```python
from build123d import *

# Parameters (mm, degrees)
CROQUIS1_R              = 4
SALIENTE_EXTRUIR1_DEPTH = 171
CROQUIS2_R              = 17.5
SALIENTE_EXTRUIR2_DEPTH = 3
SALIENTE_EXTRUIR3_DEPTH = 5
CROQUIS4_R              = 4
SALIENTE_EXTRUIR4_DEPTH = 4.5
CROQUIS8_R              = 17.5
SALIENTE_EXTRUIR6_DEPTH = 3


with BuildPart() as part:
    # Croquis1 → Saliente-Extruir1 (new body)
    with BuildSketch(Plane(origin=(0, 0, 0), x_dir=(1, 0, 0), z_dir=(0, 1, 0))):
        Circle(CROQUIS1_R)
    extrude(amount=SALIENTE_EXTRUIR1_DEPTH)

    # Croquis2 → Saliente-Extruir2 (add)
    with BuildSketch(Plane(origin=(0, 29.389431256, -17.658951857), x_dir=(-1, 0, 0), z_dir=(0, -0.857167301, 0.515038075))):
        with Locations((0, -20.601522996)):
            Circle(CROQUIS2_R)
    extrude(amount=SALIENTE_EXTRUIR2_DEPTH)

    # Croquis3 → Saliente-Extruir3 (add)
    with BuildSketch(Plane(origin=(0, 171, 0), x_dir=(1, 0, 0), z_dir=(0, 1, 0))):
        with BuildLine():
            Line((1.050742858, 12.216507919), (0.472845286, 10.71499343))
            ThreePointArc((0.472845286, 10.71499343), (0, 10.543875222), (-0.472845286, 10.71499343))
            Line((-0.472845286, 10.71499343), (-1.050742858, 12.216507919))
            ThreePointArc((-1.050742858, 12.216507919), (-1.656207782, 12.14924286), (-2.257584572, 12.051988972))
            Line((-2.257584572, 12.051988972), (-2.426564451, 10.457781423))
            ThreePointArc((-2.426564451, 10.457781423), (-2.771930057, 10.239934406), (-3.179948954, 10.255912654))
            Line((-3.179948954, 10.255912654), (-4.120766374, 11.54843759))
            ThreePointArc((-4.120766374, 11.54843759), (-4.690827714, 11.328868507), (-5.249245828, 11.081179745))
            Line((-5.249245828, 11.081179745), (-5.000525386, 9.501805204))
            ThreePointArc((-5.000525386, 9.501805204), (-5.277739988, 9.201993948), (-5.675991453, 9.111824689))
            Line((-5.675991453, 9.111824689), (-6.923284582, 10.120042336))
            ThreePointArc((-6.923284582, 10.120042336), (-7.417219229, 9.763809974), (-7.892857245, 9.383492462))
            Line((-7.892857245, 9.383492462), (-7.239355878, 7.912212973))
            ThreePointArc((-7.239355878, 7.912212973), (-7.429527758, 7.55086912), (-7.790871612, 7.360697239))
            Line((-7.790871612, 7.360697239), (-9.275101788, 8.019950942))
            ThreePointArc((-9.275101788, 8.019950942), (-9.658562641, 7.553760256), (-10.018615343, 7.069262543))
            Line((-10.018615343, 7.069262543), (-8.990483327, 5.797332815))
            ThreePointArc((-8.990483327, 5.797332815), (-9.080652586, 5.39908135), (-9.380463842, 5.121866748))
            Line((-9.380463842, 5.121866748), (-11.018384727, 5.379807088))
            ThreePointArc((-11.018384727, 5.379807088), (-11.266454067, 4.838815873), (-11.487980236, 4.286424664))
            Line((-11.487980236, 4.286424664), (-10.134571292, 3.301290316))
            ThreePointArc((-10.134571292, 3.301290316), (-10.118593045, 2.893271419), (-10.336440061, 2.547905812))
            Line((-10.336440061, 2.547905812), (-12.0307187, 2.368318783))
            ThreePointArc((-12.0307187, 2.368318783), (-12.129855039, 1.792691558), (-12.201465745, 1.212996274))
            Line((-12.201465745, 1.212996274), (-10.593652069, 0.594186647))
            ThreePointArc((-10.593652069, 0.594186647), (-10.472615206, 0.204206132), (-10.593652069, -0.185774383))
            Line((-10.593652069, -0.185774383), (-12.234346993, -0.817239228))
            ThreePointArc((-12.234346993, -0.817239228), (-12.183011813, -1.386127504), (-12.105238209, -1.952007737))
            Line((-12.105238209, -1.952007737), (-10.336440061, -2.139493548))
            ThreePointArc((-10.336440061, -2.139493548), (-10.118593045, -2.484859155), (-10.134571292, -2.892878051))
            Line((-10.134571292, -2.892878051), (-11.603765461, -3.962291436))
            ThreePointArc((-11.603765461, -3.962291436), (-11.411733847, -4.485471759), (-11.196127365, -4.999385795))
            Line((-11.196127365, -4.999385795), (-9.380463842, -4.713454484))
            ThreePointArc((-9.380463842, -4.713454484), (-9.080652586, -4.990669086), (-8.990483327, -5.388920551))
            Line((-8.990483327, -5.388920551), (-10.170571543, -6.848839375))
            ThreePointArc((-10.170571543, -6.848839375), (-9.857154436, -7.29271093), (-9.524379813, -7.722261033))
            Line((-9.524379813, -7.722261033), (-7.790871612, -6.952284975))
            ThreePointArc((-7.790871612, -6.952284975), (-7.429527758, -7.142456856), (-7.239355878, -7.503800709))
            Line((-7.239355878, -7.503800709), (-8.024406446, -9.271247353))
            ThreePointArc((-8.024406446, -9.271247353), (-7.61599094, -9.60956858), (-7.193327687, -9.929912542))
            Line((-7.193327687, -9.929912542), (-5.675991453, -8.703412424))
            ThreePointArc((-5.675991453, -8.703412424), (-5.277739988, -8.793581684), (-5.000525386, -9.09339294))
            Line((-5.000525386, -9.09339294), (-5.309068741, -11.052642915))
            ThreePointArc((-5.309068741, -11.052642915), (-4.836465093, -11.26746341), (-4.355191926, -11.462086615))
            Line((-4.355191926, -11.462086615), (-3.179948954, -9.84750039))
            ThreePointArc((-3.179948954, -9.84750039), (-2.771930057, -9.831522142), (-2.426564451, -10.049369159))
            Line((-2.426564451, -10.049369159), (-2.213426541, -12.060176999))
            ThreePointArc((-2.213426541, -12.060176999), (-1.70946512, -12.141863749), (-1.202540078, -12.202500713))
            Line((-1.202540078, -12.202500713), (-0.472845286, -10.306581166))
            ThreePointArc((-0.472845286, -10.306581166), (-0.08286477, -10.185544303), (0.307115745, -10.306581166))
            Line((0.307115745, -10.306581166), (1.042474215, -12.217216287))
            ThreePointArc((1.042474215, -12.217216287), (1.544818551, -12.163908169), (2.04454079, -12.08995365))
            Line((2.04454079, -12.08995365), (2.26083491, -10.049369159))
            ThreePointArc((2.26083491, -10.049369159), (2.606200516, -9.831522142), (3.014219413, -9.84750039))
            Line((3.014219413, -9.84750039), (4.224886916, -11.510753965))
            ThreePointArc((4.224886916, -11.510753965), (4.693799885, -11.327637394), (5.154801423, -11.125428018))
            Line((5.154801423, -11.125428018), (4.834795845, -9.09339294))
            ThreePointArc((4.834795845, -9.09339294), (5.112010447, -8.793581684), (5.510261912, -8.703412424))
            Line((5.510261912, -8.703412424), (7.105542644, -9.992916993))
            ThreePointArc((7.105542644, -9.992916993), (7.511283882, -9.691632511), (7.90426552, -9.37388462))
            Line((7.90426552, -9.37388462), (7.073626337, -7.503800709))
            ThreePointArc((7.073626337, -7.503800709), (7.263798217, -7.142456856), (7.625142071, -6.952284975))
            Line((7.625142071, -6.952284975), (9.480310931, -7.776299309))
            ThreePointArc((9.480310931, -7.776299309), (9.796043302, -7.374595712), (10.094766478, -6.960087359))
            Line((10.094766478, -6.960087359), (8.824753786, -5.388920551))
            ThreePointArc((8.824753786, -5.388920551), (8.914923046, -4.990669086), (9.214734302, -4.713454484))
            Line((9.214734302, -4.713454484), (11.185209251, -5.023765551))
            ThreePointArc((11.185209251, -5.023765551), (11.388040568, -4.545289685), (11.570414703, -4.058648777))
            Line((11.570414703, -4.058648777), (9.968841751, -2.892878051))
            ThreePointArc((9.968841751, -2.892878051), (9.952863504, -2.484859155), (10.17071052, -2.139493548))
            Line((10.17071052, -2.139493548), (12.108106386, -1.934137026))
            ThreePointArc((12.108106386, -1.934137026), (12.180495026, -1.408072161), (12.230038474, -0.879366378))
            Line((12.230038474, -0.879366378), (10.427922528, -0.185774383))
            ThreePointArc((10.427922528, -0.185774383), (10.306885665, 0.204206132), (10.427922528, 0.594186647))
            Line((10.427922528, 0.594186647), (12.195208041, 1.274373229))
            ThreePointArc((12.195208041, 1.274373229), (12.12666239, 1.8141625), (12.034236318, 2.350379234))
            Line((12.034236318, 2.350379234), (10.17071052, 2.547905812))
            ThreePointArc((10.17071052, 2.547905812), (9.952863504, 2.893271419), (9.968841751, 3.301290316))
            Line((9.968841751, 3.301290316), (11.452232826, 4.381037502))
            ThreePointArc((11.452232826, 4.381037502), (11.241020253, 4.897610638), (11.006520824, 5.404037901))
            Line((11.006520824, 5.404037901), (9.214734302, 5.121866748))
            ThreePointArc((9.214734302, 5.121866748), (8.914923046, 5.39908135), (8.824753786, 5.797332815))
            Line((8.824753786, 5.797332815), (9.940895623, 7.178141856))
            ThreePointArc((9.940895623, 7.178141856), (9.595346713, 7.633901214), (9.228920544, 8.073050965))
            Line((9.228920544, 8.073050965), (7.625142071, 7.360697239))
            ThreePointArc((7.625142071, 7.360697239), (7.263798217, 7.55086912), (7.073626337, 7.912212973))
            Line((7.073626337, 7.912212973), (7.77177818, 9.48401762))
            ThreePointArc((7.77177818, 9.48401762), (7.310768329, 9.843769234), (6.83313078, 10.181132061))
            Line((6.83313078, 10.181132061), (5.510261912, 9.111824689))
            ThreePointArc((5.510261912, 9.111824689), (5.112010447, 9.201993948), (4.834795845, 9.501805204))
            Line((4.834795845, 9.501805204), (5.094829592, 11.15301922))
            ThreePointArc((5.094829592, 11.15301922), (4.547139411, 11.387302116), (3.988716959, 11.594708419))
            Line((3.988716959, 11.594708419), (3.014219413, 10.255912654))
            ThreePointArc((3.014219413, 10.255912654), (2.606200516, 10.239934406), (2.26083491, 10.457781423))
            Line((2.26083491, 10.457781423), (2.088629995, 12.082414951))
            ThreePointArc((2.088629995, 12.082414951), (1.571117662, 12.16053928), (1.050742858, 12.216507919))
        make_face()
    extrude(amount=SALIENTE_EXTRUIR3_DEPTH)

    # Croquis4 → Saliente-Extruir4 (add)
    with BuildSketch(Plane(origin=(0, 176, 0), x_dir=(1, 0, 0), z_dir=(0, 1, 0))):
        Circle(CROQUIS4_R)
    extrude(amount=SALIENTE_EXTRUIR4_DEPTH)

    # Croquis8 → Saliente-Extruir6 (add)
    with BuildSketch(Plane(origin=(0, 102.863009395, 61.8063315), x_dir=(-1, 0, 0), z_dir=(0, 0.857167301, 0.515038075))):
        with Locations((0, -72.105330487)):
            Circle(CROQUIS8_R)
    extrude(amount=SALIENTE_EXTRUIR6_DEPTH)


solid = part.part
```
The model under review builds one solid part; all positions refer to its coordinate system, in mm. A direction names the side the tool comes from. Give positions to 0.01 mm unless a question says otherwise; leave off trailing zeros. Write each loop counter-clockwise with the first axis right and the second up, starting at its lowest first coordinate (ties: lowest second). Pieces come first, ordered by that corner, then holes. Notation, with made-up numbers: (10.25, -7) -> (22.25, -7) arc R33 cw to (22.25, 27) -> close; hole circle Ø11 at (51, -14.75). An arc over 180 degrees is marked (long way). Answer in a Markdown table with one row per item.
1) For L1, parallel to Y at x = 3, z = -6.5; L2, parallel to Y at x = -7, z = 3; L3, parallel to X at y = 97, z = -0.5, list the stretches that pass through material, from the lowest coordinate up. Write a range as [from, to].
Worked answers:
| item | result |
|---|---|
| L1 | [32.59, 36.09], [143.91, 147.41], [171, 176] |
| L2 | [38.3, 41.8], [138.2, 141.7], [171, 176] |
| L3 | [-3.97, 3.97] |
2) Clearance check with flat-ended pins moving along their axes: P1, Ø12, axis at x = -4, y = 75.5, coming from the +Z side; P2, Ø6, axis at y = 71.5, z = 6.5, coming from the +X side; P3, Ø1.5, axis at y = 28, z = 0, coming from the +X side; P4, Ø7.5, axis at x = -4.5, z = -1.5, coming from the +Y side. State where each tip first meets the part, or that it passes through.
Worked answers:
| item | result |
|---|---|
| P1 | z = 4 |
| P2 | x = 1.94 |
| P3 | x = 4 |
| P4 | y = 180.5 |
3) Add section A-A on y = 69. State the section outline as (x, z) points.
Worked answers:
| item | result |
|---|---|
| outline | circle Ø8 at (0, 0) |
4) Tool access review of faces 1 (the flat face through (0, 180.5, 0)), 2 (the cylindrical face through (-0.867, 19.179, 3.905)), 3 (the cylindrical face through (-0.867, 89.237, 3.905)), 4 (the flat face through (0, 0, 0)), 5 (the flat face through (-3, 176, -3)): name each direction out of +Z, -Z, +X, -X, +Y, -Y from which nothing blocks a thin tool from reaching the whole face with its end or side.
Worked answers:
| item | result |
|---|---|
| face 1 | +Z, -Z, +X, -X, +Y |
| face 2 | -Y |
| face 3 | none |
| face 4 | +Z, -Z, +X, -X, -Y |
| face 5 | +Y |
